Verification items for the finished model (mm, model axes). A direction names the side the tool comes from. Coordinates: 2 decimals unless noted, no trailing zeros. Order: outer loops, then holes, each group sorted by start corner. A loop starts at its lowest first (then second) coordinate and runs counter-clockwise, first axis right, second up. Notation, with made-up numbers: (44.25, 57.25) -> (77.25, 57.25) arc R16 cw to (77.25, 83.25) -> close; hole circle Ø5 at (23.5, -10). An arc over 180 degrees is marked (long way). Write item = value, one per line. Start each with the question number.
1. Set-up check for faces 1 (the flat face through (-10, 6, -23)), 2 (the flat face through (110, 6, 1)): record each of +Z, -Z, +X, -X, +Y, -Y from which the full face is reachable in a straight line by a thin tool's end or side.
2. Release check for a two-part mould opening along Z. For faces 3 (the cylindrical face through (-113.145, 6.084, 85.173)), 4 (the flat face through (-14, 6, -90)), 5 (the flat face through (13, 0, -21)) record: +Z half, -Z half, draft (parallel to the pull), parting line (faces both ways), or undercut.
3. Cross-section at B-B on x = 89. Record the cut outline in (y, z), plus the area to 3 significant figures.
4. Thickness scan on line 1 along X through (y, z) = (6.25, -80); line 2 along X through (y, z) = (3.25, 80); line 3 along X through (y, z) = (5.25, 0). Record the ranges inside material, lowest first. Write a range as from..to.
5. Cross-section at C-C on x = -70. Record the cut outline in (y, z).
6. Cross-section at D-D on y = 10. Give the number of separate pieces and of enclosed holes in the cut face, plus the area to 3 significant figures.
7. Go/stop test with a flat-tipped pin: P1, Ø8, axis at x = -116.53, z = -45.39, coming from the +Y side. Record where the tip stops, or that it passes through.
8. Cross-section at A-A on z = 0. Record the cut outline in (x, y), plus the area to 3 significant figures.
from build123d import *

# Parameters (mm, degrees)
SKETCH1_W                 = 245
SKETCH1_H                 = 180
BOSS_EXTRUDE1_DEPTH       = 12
CHAMFER2_SIZE             = 4
M8_TAPPED_HOLE1_D         = 6.8
M6_TAPPED_HOLE1_D         = 5
CHAMFER3_SIZE             = 1
SKETCH_PATTERN1_OUTLINE_R = 2.5
SKETCH_PATTERN1_DEPTH     = 12
SKETCH_PATTERN2_OUTLINE_R = 3.4
SKETCH_PATTERN2_DEPTH     = 12
CUT_EXTRUDE1_REACH        = 164.693
SKETCH11_R                = 5.6
SKETCH_PATTERN4_OUTLINE_R = 3.9
SKETCH_PATTERN4_DEPTH     = 12


# Read off the part's stored shape, not the designer's step: Sketch-Pattern1, Sketch-Pattern2, Sketch-Pattern4
with BuildPart() as part:
    # Sketch1 → Boss-Extrude1 (new body)
    with BuildSketch(Plane(origin=(0, 0, 0), x_dir=(1, 0, 0), z_dir=(0, 1, 0))):
        with Locations((-12.5, 0)):
            Rectangle(SKETCH1_W, SKETCH1_H)
        with BuildLine():
            Line((0, 23), (-20.040016013, 23))
            ThreePointArc((-20.040016013, 23), (-125, 0), (-20.040016013, -23))
            Line((-20.040016013, -23), (0, -23))
            ThreePointArc((0, -23), (23, 0), (0, 23))
        make_face(mode=Mode.SUBTRACT)
    extrude(amount=BOSS_EXTRUDE1_DEPTH)

    # Chamfer2
    chamfer2_edges = [part.edges().sort_by_distance(p)[0] for p in [
        (-135, 6, -90),
        (110, 6, -90),
        (110, 6, 90),
        (-135, 6, 90),
    ]]
    chamfer(chamfer2_edges, length=CHAMFER2_SIZE)

    # M8 Tapped Hole1 (through all)
    with Locations(Plane(origin=(0, 12, 0), x_dir=(1, 0, 0), z_dir=(0, 1, 0))):
        with Locations((-115.961940777, -45.961940777)):
            Hole(M8_TAPPED_HOLE1_D / 2)

    # M6 Tapped Hole1 (through all)
    with Locations(Plane(origin=(0, 12, 0), x_dir=(1, 0, 0), z_dir=(0, 1, 0))):
        with Locations((0, 33)):
            Hole(M6_TAPPED_HOLE1_D / 2)

    # Chamfer3
    chamfer3_edges = [part.edges().sort_by_distance(p)[0] for p in [
        (23, 0, 0),
        (-10.020008006, 0, -23),
        (-125, 0, 0),
        (-10.020008006, 0, 23),
    ]]
    chamfer(chamfer3_edges, length=CHAMFER3_SIZE)

    # Sketch-Pattern1 outline → Sketch-Pattern1 (cut)
    with BuildSketch(Plane(origin=(0, 0, 0), x_dir=(1, 0, 0), z_dir=(0, 1, 0))):
        with Locations((0, -33)):
            Circle(SKETCH_PATTERN1_OUTLINE_R)
        with Locations((33, 0)):
            Circle(SKETCH_PATTERN1_OUTLINE_R)
    extrude(amount=SKETCH_PATTERN1_DEPTH, mode=Mode.SUBTRACT)

    # Sketch-Pattern2 outline → Sketch-Pattern2 (cut)
    with BuildSketch(Plane(origin=(0, 0, 0), x_dir=(1, 0, 0), z_dir=(0, 1, 0))):
        with Locations((-116.529552601, 45.387230966)):
            Circle(SKETCH_PATTERN2_OUTLINE_R)
        with Locations((-24.038059223, 45.961940777)):
            Circle(SKETCH_PATTERN2_OUTLINE_R)
        with Locations((-23.470447399, -45.387230966)):
            Circle(SKETCH_PATTERN2_OUTLINE_R)
    extrude(amount=SKETCH_PATTERN2_DEPTH, mode=Mode.SUBTRACT)

    # Sketch11 → Cut-Extrude1 (cut, up to next)
    with BuildSketch(Plane(origin=(0, 12, 0), x_dir=(1, 0, 0), z_dir=(0, 1, 0)), mode=Mode.PRIVATE) as cut_extrude1_sk1:
        with Locations(Location((-111, -80, 0), (0, 0, 270))):
            Circle(SKETCH11_R)
    cut_extrude1_tool1 = extrude(cut_extrude1_sk1.sketch, amount=-CUT_EXTRUDE1_REACH, mode=Mode.PRIVATE) & part.part
    cut_extrude1 = cut_extrude1_tool1.solids().sort_by_distance((-111, 12, 80))[0]
    add(cut_extrude1, mode=Mode.SUBTRACT)

    # Sketch-Pattern3: Cut-Extrude1 at 3 more places
    with Locations((200, 0, 0), (200, 0, -160), (0, 0, -160)):
        add(cut_extrude1, mode=Mode.SUBTRACT)

    # Sketch-Pattern4 outline → Sketch-Pattern4 (cut)
    with BuildSketch(Plane(origin=(0, 0, 0), x_dir=(1, 0, 0), z_dir=(0, 1, 0))):
        with Locations((-81, -80)):
            Circle(SKETCH_PATTERN4_OUTLINE_R)
        with Locations((59, 80)):
            Circle(SKETCH_PATTERN4_OUTLINE_R)
    extrude(amount=SKETCH_PATTERN4_DEPTH, mode=Mode.SUBTRACT)


solid = part.part
Worked out:
q1.face_1 = +Y, -Y
q1.face_2 = +Z, -Z, +X, +Y, -Y
q2.face_3 = undercut
q2.face_4 = -Z half
q2.face_5 = draft
q3.outline = (0, -90) -> (12, -90) -> (12, -85.6) -> (0, -85.6) -> close; (0, -74.4) -> (12, -74.4) -> (12, 74.4) -> (0, 74.4) -> close; (0, 85.6) -> (12, 85.6) -> (12, 90) -> (0, 90) -> close
q3.area = 1,890 mm²
q4.line_1 = -135..-116.6, -105.4..55.1, 62.9..83.4, 94.6..110
q4.line_2 = -135..-116.6, -105.4..-84.9, -77.1..83.4, 94.6..110
q4.line_3 = -135..-125, 23..30.5, 35.5..110
q5.outline = (0, -90) -> (12, -90) -> (12, -55) -> (1, -55) -> (0, -56) -> close; (0, 56) -> (1, 55) -> (12, 55) -> (12, 90) -> (0, 90) -> close
q6.separate_pieces = 1
q6.enclosed_holes = 14
q6.area = 32,300 mm²
q7.P1 = 12
q8.outline = (-135, 0) -> (-126, 0) -> (-125, 1) -> (-125, 12) -> (-135, 12) -> close; (23, 1) -> (24, 0) -> (30.5, 0) -> (30.5, 12) -> (23, 12) -> close; (35.5, 0) -> (110, 0) -> (110, 12) -> (35.5, 12) -> close
q8.area = 1,100 mm²
